Autodesk Inventor part; units mm, degrees
ref_plane "Work Plane1" through (0, 0, 2.75) normal (0, 0, 1) x (1, 0, 0)
ref_plane "Work Plane3" through (7.0312, 0, 0) normal (0, 1, 0) x (-1, 0, 0)
ref_plane "YZ Plane" through (0, 0, 0) normal (1, 0, 0) x (0, 1, 0)
sketch "Sketch1" plane through (0, 0, 0) normal (1, 0, 0) x (0, 1, 0)
  circle A0 centre (0, 0) radius 2.75
  dimension "d0" = 5.5
extrude "Body" add sketch "Sketch1" along normal mid plane 2
sketch "Sketch2" plane through (-1, 0, 0) normal (-1, 0, 0) x (0, 0, 1)
  line L0 (0, -3.85) -> (0, 3.85)
  line L1 (-3.85, 0) -> (3.85, 0)
  point P0 (0, 0)
  point P1 (0, 0)
hole "Thread" at (-1, 0, 0) direction (1, 0, 0) diameter 1.567 end through all
ref_plane "Work Plane1" through (0, 0, 2.75) normal (0, 0, 1) x (1, 0, 0)
sketch "Sketch3" plane through (0, 0, 2.75) normal (0, 0, 1) x (1, 0, 0)
  line L0 (-1.4, 0) -> (1.4, 0)
  line L1 (0, 3.85) -> (0, -3.85)
  point P0 (0, 0)
hole "Hole" at (0, 0, 2.75) direction (0, 0, -1) diameter 1 depth 1.4 tip angle 120
pattern_circular "Holes" count 4 over 360 about axis through (-10, 0, 0) along (1, 0, 0) of "Hole"
chamfer "Chamfer1" distance 0.2 angle 45 1 edges at (-1, -2.75, 0) measured on face at (-0.0044, -2.5506, 1.028)
chamfer "Chamfer2" distance 0.2 angle 45 1 edges at (1, -2.75, 0) measured on face at (0.0623, -2.5506, 1.028)
chamfer "Chamfer3" distance 0.2165 angle 30 1 edges at (-1, 0, -0.7835) measured on face at (-1, 1.9346, -0.2349)
ref_plane "Work Plane3" through (7.0312, 0, 0) normal (0, 1, 0) x (-1, 0, 0)
equation "\"d0\" = SD2"
equation "\"d1\" = KOH"
equation "\"d7\" = BOR"
equation "\"d9\" = ANG"
equation "\"d8\" = LOTI"
equation "\"d3\" = PHH1"
equation "\"d61\" = PHH1"
equation "\"d5\" = PHH"
equation "\"d62\" = PHH"
equation "\"d12\" = -0.5 * GD1 + 0.5 * NND"
equation "\"d63\" = -0.5 * GD1 + 0.5 * NND"
equation "\"FAWI1\" = 45deg"
equation "\"FAWI\" = 45deg"
equation "\"ANG\" = 120deg"
equation "\"NND\" = 2"
equation "\"KOH\" = 2"
equation "\"SD2\" = 5.5"
equation "\"BOR\" = 1"
equation "\"LOTI\" = 1.4"
equation "\"PHH\" = 0.2"
equation "\"PHH1\" = PHH"
equation "\"GUL\" = 0.541266 * PTC"
equation "\"THREADDIA\" = 2"
equation "\"PTC\" = 0.4"
equation "\"GAL\" = 0.541266 * PTC"
equation "\"TOA\" = 30deg"
properties part number "CNS 4433 - M 2" material "Steel, Mild"
The model under review builds one solid part; all positions refer to its coordinate system, in mm. A direction names the side the tool comes from. Coordinates: 2 decimals unless noted, no trailing zeros. Write each loop counter-clockwise with the first axis right and the second up, starting at its lowest first coordinate (ties: lowest second). Pieces come first, ordered by that corner, then holes. Notation, with made-up numbers: (72.5, 39) - (100.5, 39) arc R16 cw to (100.5, 60) - close; hole circle Ø10 at (-10, 19). An arc over 180 degrees is marked (long way). Write item = value, one per line.
(1) Consider section A-A, the plane x = 0.65. Give the boundary of the cut face in (y, z).
Result sheet:
outline = circle Ø5.5 at (0, 0); hole circle Ø1.57 at (0, 0)
(2) For line 1 (X direction, y = 0, z = -2); line 2 (Z direction, x = 0.55, y = 0); line 3 (Z direction, x = 0, y = -2.15), list the stretches that pass through material, from the lowest coordinate up. Write a range as [from, to].
Result sheet:
line_1 = [-1, -0.5], [0.5, 1]
line_2 = [-2.75, -0.78], [0.78, 2.75]
line_3 = [-1.71, -0.5], [0.5, 1.71]
(3) Mouldability with a two-part tool opening along X and no side actions: class faces 1 (the face through (0.076, -0.235, 0.747)), 2 (the face through (-1, 1, -1)), 3 (the face through (0.488, -0.108, -2.04)) as pulls with the +X half, pulls with the -X half, needs draft (parallel to the pull), parting line crosses it, or undercut.
Result sheet:
face_1 = needs draft
face_2 = pulls with the -X half
face_3 = undercut
(4) Machinability: for faces 4 (the face through (1, 1, 1)), 5 (the face through (0.488, -2.04, 0.108)), 6 (the face through (0.488, 0.108, 2.04)), 7 (the face through (0.488, 2.04, -0.108)), which of the approach directions +Z, -Z, +X, -X, +Y, -Y give a long, thin tool a straight path to every point of the face, cutting with its end or side? Answer none if there is none.
Result sheet:
face_4 = +Z, -Z, +X, +Y, -Y
face_5 = -Y
face_6 = +Z
face_7 = +Y
